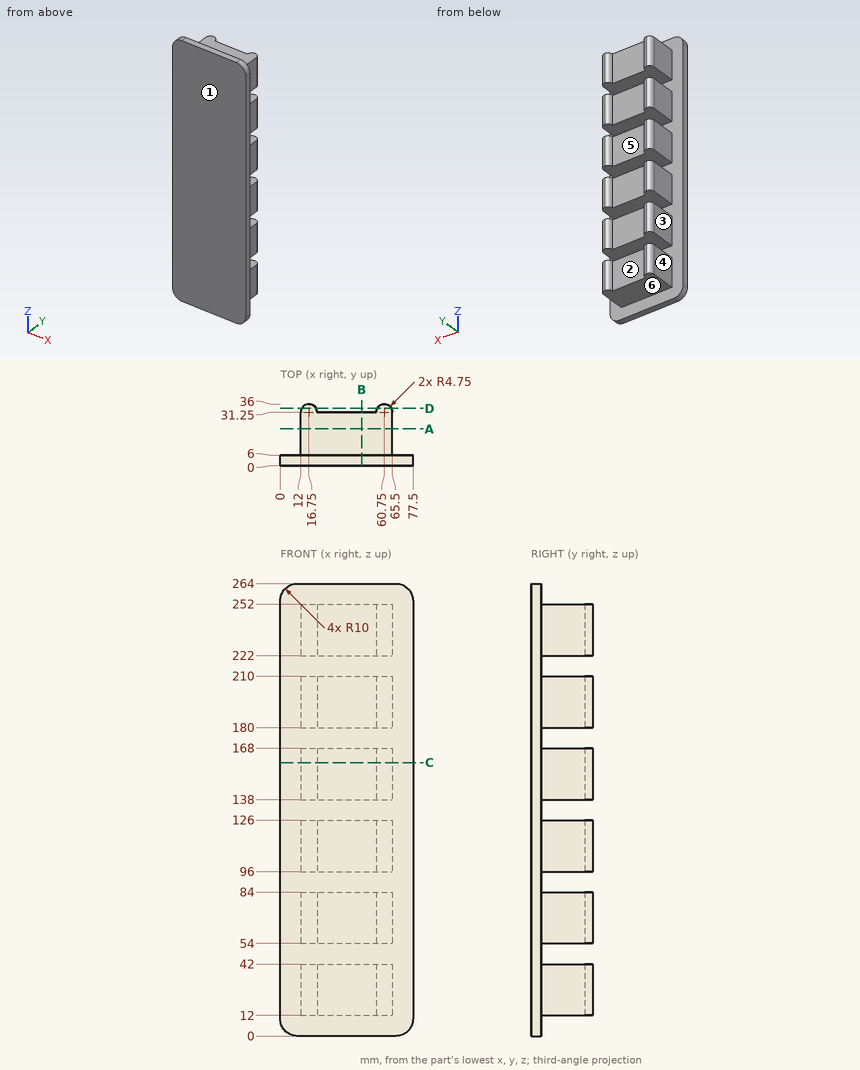
Study the drawing (mm; zero at the part's minimum x, y, z) and answer. A direction names the side the tool comes from. Coordinates: 2 decimals unless noted, no trailing zeros. Write each loop counter-clockwise with the first axis right and the second up, starting at its lowest first coordinate (ties: lowest second). Pieces come first, ordered by that corner, then holes. Notation, with made-up numbers: M 27,73 L 45,73 A31 cw 45,105 Z; hole C 9,-21.75 d8. An arc over 180 degrees is marked long. Use a Markdown table: item, result. Add a question column.
1. Straight lines are drawn through the part: line 1 along Z through (x, y) = (45, 31); line 2 along Y through (x, z) = (25, 207); line 3 along Y through (x, z) = (68, 238). For each, find the intervals that lie inside material, in ascending order. Write a range as [from, to].
2. For a pull along X with two mould halves and no side action, classify the marked faces 1, 2 and 3 as +X half, -X half, draft (parallel to the pull), parting line (faces both ways), or undercut.
3. Section D-D (y = 33.5) is taken. Count the separate pieces of the cut face and the enclosed holes in it, plus the area to 3 significant figures.
4. Which of the six approach directions +Z, -Z, +X, -X, +Y, -Y give full straight-line access (tool end or side, diameter ignored) to the marked faces 4, 5 and 6?
5. Given P1, Ø5, axis at x = 33.5, y = 10.5, coming from the -Z side; P2, Ø15, axis at x = 42, y = 26.5, coming from the +Z side; P3, Ø4, axis at y = 20, z = 35.5, coming from the +X side; P4, Ø3, axis at x = 33.5, z = 230.5, coming from the -Y side, each flat-ended and moving along its own axis, determine where each tip first touches the part or whether it passes through.
6. Section A-A (y = 21.5) is taken. Give the vertices of the cut face in (x, z).
7. Section C-C (z = 159.5) is taken. Give the vertices of the cut face in (x, y).
8. Section B-B (x = 47.5) is taken. Give the vertices of the cut face in (y, z).
Data:
| question | item | result |
|---|---|---|
| 1 | line 1 | z = [12, 42], [54, 84], [96, 126], [138, 168], [180, 210], [222, 252] |
| 1 | line 2 | y = [0, 31.25] |
| 1 | line 3 | y = [0, 6] |
| 2 | face 1 | draft |
| 2 | face 2 | undercut |
| 2 | face 3 | -X half |
| 3 | separate pieces | 12 |
| 3 | enclosed holes | 0 |
| 3 | area | 3,010 mm2 |
| 4 | face 4 | +Z, -Z, -X, +Y |
| 4 | face 5 | +Z, -Z, +Y |
| 4 | face 6 | -Z, +X, -X, +Y |
| 5 | P1 | stops at z = 12 |
| 5 | P2 | stops at z = 252 |
| 5 | P3 | stops at x = 65.5 |
| 5 | P4 | stops at y = 0 |
| 6 | outline | M 12,12 L 65.5,12 L 65.5,42 L 12,42 Z; M 12,54 L 65.5,54 L 65.5,84 L 12,84 Z; M 12,96 L 65.5,96 L 65.5,126 L 12,126 Z; M 12,138 L 65.5,138 L 65.5,168 L 12,168 Z; M 12,180 L 65.5,180 L 65.5,210 L 12,210 Z; M 12,222 L 65.5,222 L 65.5,252 L 12,252 Z |
| 7 | outline | M 0,0 L 77.5,0 L 77.5,6 L 65.5,6 L 65.5,31.25 A4.75 ccw 56,31.25 L 21.5,31.25 A4.75 ccw 12,31.25 L 12,6 L 0,6 Z |
| 8 | outline | M 0,0 L 6,0 L 6,12 L 31.25,12 L 31.25,42 L 6,42 L 6,54 L 31.25,54 L 31.25,84 L 6,84 L 6,96 L 31.25,96 L 31.25,126 L 6,126 L 6,138 L 31.25,138 L 31.25,168 L 6,168 L 6,180 L 31.25,180 L 31.25,210 L 6,210 L 6,222 L 31.25,222 L 31.25,252 L 6,252 L 6,264 L 0,264 Z |
